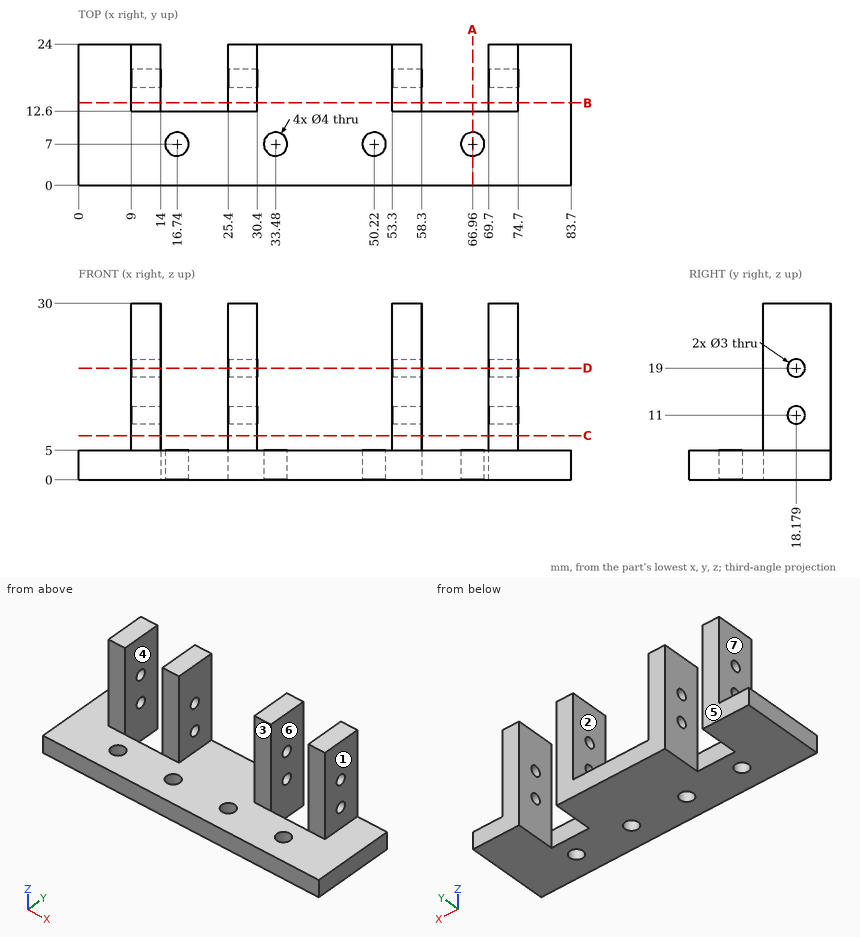
Input: dimensioned drawing with shaded views. Units: mm. Origin: part minimum x, y, z. A direction names the side the tool comes from. Give positions to 0.01 mm unless a question says otherwise; leave off trailing zeros. Write each loop counter-clockwise with the first axis right and the second up, starting at its lowest first coordinate (ties: lowest second). Pieces come first, ordered by that corner, then holes. Notation, with made-up numbers: (-16, -11.75) -> (2, -11.75) arc R22 ccw to (2, 11.25) -> close; hole circle Ø10 at (-29, -3.5). An arc over 180 degrees is marked (long way). Answer as a JSON object with one key per item and string values.
1. Cut plane B-B on y = 14. Output: boundary loops of the cut face in (x, z).
Ans:
{"outline": "(0, 0) -> (14, 0) -> (14, 30) -> (9, 30) -> (9, 5) -> (0, 5) -> close; (25.4, 0) -> (58.3, 0) -> (58.3, 30) -> (53.3, 30) -> (53.3, 5) -> (30.4, 5) -> (30.4, 30) -> (25.4, 30) -> close; (69.7, 0) -> (83.7, 0) -> (83.7, 5) -> (74.7, 5) -> (74.7, 30) -> (69.7, 30) -> close"}
2. Ray query, probe 1 along X at (y, z) = (23, 22); probe 2 along Z at (x, y) = (7, 14.25); probe 3 along Y at (x, z) = (57, 6.75). Return the intervals inside material, ascending. Write a range as from..to.
Ans:
{"probe 1": "x = 9..14, 25.4..30.4, 53.3..58.3, 69.7..74.7", "probe 2": "z = 0..5", "probe 3": "y = 12.6..24"}
3. Contact query for flat-ended pins moving along their axis: pin 1 (1.5 mm diameter, centred on x = 37.5, y = 15, fed in from +Z); pin 2 (4 mm diameter, centred on x = 71.5, z = 22, fed in from -Y); pin 3 (1.8 mm diameter, centred on y = 18.18, z = 11, fed in from +X); pin 4 (9 mm diameter, centred on y = 18.5, z = 16, fed in from +X). Output: stop coordinate, or through.
Ans:
{"pin 1": "stops at z = 5", "pin 2": "stops at y = 12.6", "pin 3": "passes through", "pin 4": "stops at x = 74.7"}
4. Cut plane C-C on z = 7.5. Output: boundary loops of the cut face in (x, y).
Ans:
{"outline": "(9, 12.6) -> (14, 12.6) -> (14, 24) -> (9, 24) -> close; (25.4, 12.6) -> (30.4, 12.6) -> (30.4, 24) -> (25.4, 24) -> close; (53.3, 12.6) -> (58.3, 12.6) -> (58.3, 24) -> (53.3, 24) -> close; (69.7, 12.6) -> (74.7, 12.6) -> (74.7, 24) -> (69.7, 24) -> close"}
5. Cut plane A-A on x = 66.96. Output: boundary loops of the cut face in (y, z).
Ans:
{"outline": "(0, 0) -> (5, 0) -> (5, 5) -> (0, 5) -> close; (9, 0) -> (12.6, 0) -> (12.6, 5) -> (9, 5) -> close"}
6. Cut plane D-D on z = 19. Count the separate pieces of the cut face and the enclosed holes in it, and give its area (3 significant figures).
Ans:
{"separate pieces": "8", "enclosed holes": "0", "area": "168 mm^2"}
7. Access query for the marked faces 1, 2, 3 and 4. Directions: +Z, -Z, +X, -X, +Y, -Y. A direction counts if a zero-diameter tool reaches every point of the face in a straight line with its end or side. Return the directions, or none.
Ans:
{"face 1": "+Z, +X, +Y, -Y", "face 2": "+Z, +Y, -Y", "face 3": "+Z, +X, -X, -Y", "face 4": "+Z, -Z, +Y"}
8. Mould query, pull axis X, two halves, no side actions, for the marked faces 5, 6 and 7. Classes: pulls with the +X half, pulls with the -X half, needs draft (parallel to the pull), parting line crosses it, or undercut.
Ans:
{"face 5": "needs draft", "face 6": "undercut", "face 7": "pulls with the -X half"}
